Source: CAD feature listing. Evaluate the final solid. Frame: model axes, mm. Face numbers are marked on the shaded views. A direction names the side the tool comes from. Give positions to 0.01 mm unless a question says otherwise; leave off trailing zeros. Loops run counter-clockwise (first coordinate to the right, second up) from the corner with the lowest first, then second, coordinate; pieces in that order, holes last.
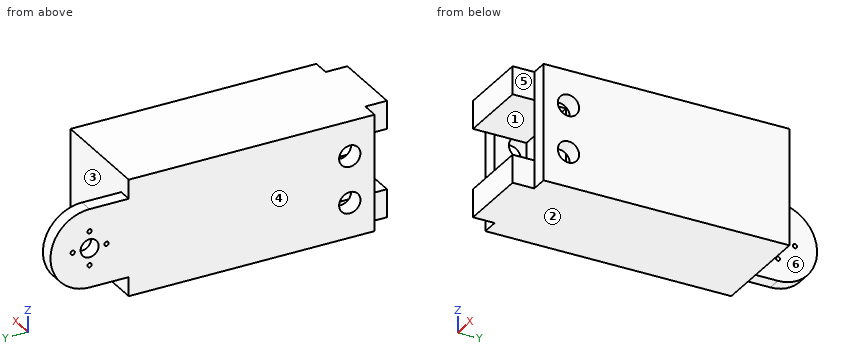
```python
from build123d import *

# Parameters (mm, degrees)
SKETCH1_W               = 50
SKETCH1_H               = 150
BOSS_EXTRUDE1_DEPTH     = 55
CUT_EXTRUDE1_DEPTH      = 168.406690428
CUT_EXTRUDE1_DEPTH_BACK = 45
SKETCH2_R               = 10.25
SKETCH7_R               = 1
SKETCH7_R_2             = 4.25
CUT_EXTRUDE3_DEPTH      = 10
SKETCH8_W               = 55
SKETCH8_H               = 55
SKETCH8_R               = 10.25
BOSS_EXTRUDE2_DEPTH     = 50
SKETCH10_W              = 8
SKETCH10_H              = 10.25
SKETCH10_W_2            = 17
SKETCH10_H_2            = 1
SKETCH10_W_3            = 34
SKETCH10_H_3            = 20
SKETCH10_H_4            = 5
CUT_EXTRUDE4_DEPTH      = 214.717102732
SKETCH11_W              = 34
SKETCH11_H              = 13.25
BOSS_EXTRUDE4_DEPTH     = 25
SKETCH13_W              = 55
SKETCH13_H              = 10
CUT_EXTRUDE5_DEPTH      = 8
SKETCH14_R              = 5.030159043
CUT_EXTRUDE6_DEPTH      = 8
SKETCH15_W              = 34
SKETCH15_H              = 0.25
BOSS_EXTRUDE5_DEPTH     = 13.25
CUT_EXTRUDE7_DEPTH      = 181.416185527
BOSS_EXTRUDE6_START     = 1.5
SKETCH19_R              = 10.25
SKETCH19_R_2            = 1
SKETCH19_R_3            = 4.25
BOSS_EXTRUDE6_DEPTH     = 1.5
CUT_EXTRUDE8_DEPTH      = 184.89467094


with BuildPart() as part:
    # Sketch1 → Boss-Extrude1 (new body)
    with BuildSketch(Plane.XY):
        with Locations((0, -75)):
            Rectangle(SKETCH1_W, SKETCH1_H)
    extrude(amount=-BOSS_EXTRUDE1_DEPTH)

    # Sketch2 → Cut-Extrude1 (cut, two sides: drawn at the far end of the back side and taken through both)
    with BuildSketch(Plane(origin=(25, 0, 0), x_dir=(0, 0, -1), z_dir=(1, 0, 0)).offset(-CUT_EXTRUDE1_DEPTH_BACK)):
        with Locations(Location((27.5, -25, 0), (0, 0, 270))):
            Circle(SKETCH2_R)
    extrude(amount=CUT_EXTRUDE1_DEPTH + CUT_EXTRUDE1_DEPTH_BACK, mode=Mode.SUBTRACT)

    # Sketch7 → Cut-Extrude3 (cut)
    with BuildSketch(Plane(origin=(-20, 0, 0), x_dir=(0, 0, -1), z_dir=(1, 0, 0))):
        with Locations(Location((27.5, -17, 0), (0, 0, 90))):
            Circle(SKETCH7_R)
        with Locations(Location((35.5, -25, 0), (0, 0, 90))):
            Circle(SKETCH7_R)
        with Locations(Location((27.5, -33, 0), (0, 0, 90))):
            Circle(SKETCH7_R)
        with Locations(Location((19.5, -25, 0), (0, 0, 90))):
            Circle(SKETCH7_R)
        with Locations(Location((27.5, -25, 0), (0, 0, 90))):
            Circle(SKETCH7_R_2)
    extrude(amount=-CUT_EXTRUDE3_DEPTH, mode=Mode.SUBTRACT)

    # Sketch8 → Boss-Extrude2 (add)
    with BuildSketch(Plane(origin=(25, 0, 0), x_dir=(0, 0, -1), z_dir=(1, 0, 0))):
        with Locations((27.5, -177.5)):
            Rectangle(SKETCH8_W, SKETCH8_H)
        with Locations(Location((27.5, -180, 0), (0, 0, 90))):
            Circle(SKETCH8_R, mode=Mode.SUBTRACT)
    extrude(amount=-BOSS_EXTRUDE2_DEPTH)

    # Sketch10 → Cut-Extrude4 (cut, through all)
    with BuildSketch(Plane.XY):
        Polygon((-17, -205), (17, -205), (17, -191.25), (0, -191.25), (-17, -191.25), align=None)
        Polygon((-25, -205), (-17, -205), (-17, -191.25), (-17, -190.25), (-25, -190.25), align=None)
        Polygon((17, -191.25), (17, -205), (25, -205), (25, -190.25), (17, -190.25), align=None)
        with Locations((-21, -185.125)):
            Rectangle(SKETCH10_W, SKETCH10_H)
        with Locations((-21, -174.875)):
            Rectangle(SKETCH10_W, SKETCH10_H)
        with Locations((21, -174.875)):
            Rectangle(SKETCH10_W, SKETCH10_H)
        with Locations((21, -185.125)):
            Rectangle(SKETCH10_W, SKETCH10_H)
        with Locations((-8.5, -185.125)):
            Rectangle(SKETCH10_W_2, SKETCH10_H)
        with Locations((8.5, -185.125)):
            Rectangle(SKETCH10_W_2, SKETCH10_H)
        Polygon((0, -180), (17, -180), (17, -169.75), (-17, -169.75), (-17, -180), align=None)
        with Locations((-8.5, -190.75)):
            Rectangle(SKETCH10_W_2, SKETCH10_H_2)
        with Locations((8.5, -190.75)):
            Rectangle(SKETCH10_W_2, SKETCH10_H_2)
        with Locations((0, -154.75)):
            Rectangle(SKETCH10_W_3, SKETCH10_H_3)
        with Locations((0, -167.25)):
            Rectangle(SKETCH10_W_3, SKETCH10_H_4)
    extrude(amount=-CUT_EXTRUDE4_DEPTH, mode=Mode.SUBTRACT)

    # Sketch11 → Boss-Extrude4 (add)
    with BuildSketch(Plane.XZ.offset(144.75)):
        with Locations((0, -6.625)):
            Rectangle(SKETCH11_W, SKETCH11_H)
        with Locations((0, -48.375)):
            Rectangle(SKETCH11_W, SKETCH11_H)
    extrude(amount=BOSS_EXTRUDE4_DEPTH)

    # Sketch13 → Cut-Extrude5 (cut)
    with BuildSketch(Plane(origin=(25, 0, 0), x_dir=(0, 0, -1), z_dir=(1, 0, 0))):
        with Locations((27.5, -164.75)):
            Rectangle(SKETCH13_W, SKETCH13_H)
    cut_extrude5 = extrude(amount=-CUT_EXTRUDE5_DEPTH, mode=Mode.SUBTRACT)

    # Mirror2: Cut-Extrude5 across plane
    add(cut_extrude5.mirror(Plane(origin=(0, 0, 0), x_dir=(0, 0, 1), z_dir=(1, 0, 0))), mode=Mode.SUBTRACT)

    # Sketch14 → Cut-Extrude6 (cut)
    with BuildSketch(Plane(origin=(25, 0, 0), x_dir=(0, 0, -1), z_dir=(1, 0, 0))):
        with Locations(Location((16.5, -148, 0), (0, 0, 90))):
            Circle(SKETCH14_R)
        with Locations(Location((38.5, -148, 0), (0, 0, 90))):
            Circle(SKETCH14_R)
    cut_extrude6 = extrude(amount=-CUT_EXTRUDE6_DEPTH, mode=Mode.SUBTRACT)

    # Mirror3: Cut-Extrude6 across plane
    add(cut_extrude6.mirror(Plane(origin=(0, 0, 0), x_dir=(0, 0, 1), z_dir=(1, 0, 0))), mode=Mode.SUBTRACT)

    # Sketch15 → Boss-Extrude5 (add)
    with BuildSketch(Plane.XY):
        with Locations((0, -169.875)):
            Rectangle(SKETCH15_W, SKETCH15_H)
    boss_extrude5 = extrude(amount=-BOSS_EXTRUDE5_DEPTH)

    # Mirror4: Boss-Extrude5 across plane
    add(boss_extrude5.mirror(Plane.XY.offset(-27.5)))

    # Sketch16 → Cut-Extrude7 (cut, through all)
    with BuildSketch(Plane.XY):
        Polygon((-18.5, 0), (-18.5, -14.75), (-18.5, -35.25), (-18.5, -43.5), (25, -43.5), (25, 0), align=None)
    extrude(amount=-CUT_EXTRUDE7_DEPTH, mode=Mode.SUBTRACT)

    # Sketch19 → Boss-Extrude6 (add)
    with BuildSketch(Plane(origin=(-20, 0, 0), x_dir=(0, 0, -1), z_dir=(1, 0, 0)).offset(BOSS_EXTRUDE6_START)):
        with Locations((27.5, -25)):
            Circle(SKETCH19_R)
        with Locations(Location((27.5, -17, 0), (0, 0, 90))):
            Circle(SKETCH19_R_2, mode=Mode.SUBTRACT)
        with Locations(Location((27.5, -33, 0), (0, 0, 90))):
            Circle(SKETCH19_R_2, mode=Mode.SUBTRACT)
        with Locations(Location((19.5, -25, 0), (0, 0, 90))):
            Circle(SKETCH19_R_2, mode=Mode.SUBTRACT)
        with Locations(Location((35.5, -25, 0), (0, 0, 90))):
            Circle(SKETCH19_R_2, mode=Mode.SUBTRACT)
        with Locations(Location((27.5, -25, 0), (0, 0, 90))):
            Circle(SKETCH19_R_3, mode=Mode.SUBTRACT)
    extrude(amount=-BOSS_EXTRUDE6_DEPTH)

    # Sketch20 → Cut-Extrude8 (cut, through all)
    with BuildSketch(Plane(origin=(-18.5, 0, 0), x_dir=(0, 0, -1), z_dir=(1, 0, 0))):
        with BuildLine():
            Line((0, 0), (0, -43.5))
            Line((0, -43.5), (9, -43.5))
            Line((9, -43.5), (9, -25))
            ThreePointArc((9, -25), (27.5, -6.5), (46, -25))
            Line((46, -25), (46, -43.5))
            Line((46, -43.5), (55, -43.5))
            Line((55, -43.5), (55, 0))
            Line((55, 0), (0, 0))
        make_face()
    extrude(amount=-CUT_EXTRUDE8_DEPTH, mode=Mode.SUBTRACT)


solid = part.part
```
(1) Section B-B, the plane x = -3. Return the cut outline in (y, z).
A:
outline: (-170, -55) - (-43.5, -55) - (-43.5, 0) - (-170, 0) - (-170, -13.25) - (-144.75, -13.25) - (-144.75, -41.75) - (-170, -41.75) - close
(2) Ray query, line 1 along Z through (x, y) = (23, -148); line 2 along Z through (x, y) = (-22.25, -25); line 3 along Y through (x, z) = (-22, -35). Return the intervals inside material, ascending.
A:
line 1: z = -55 to -43.53, -33.47 to -21.53, -11.47 to 0
line 2: z = -46 to -36.5, -34.5 to -31.75, -23.25 to -20.5, -18.5 to -9
line 3: y = -159.75 to -151.61, -144.39 to -25.87, -24.13 to -8.09
(3) Reachability of the marked faces 4, 5 and 6 from +Z, -Z, +X, -X, +Y, -Y: full face, straight path, thin tool, end or side. Return the list, or none.
A:
face 4: +Z, -Z, -X, +Y, -Y
face 5: +Z, -Z, +X, -Y
face 6: +Z, -Z, +X, +Y
(4) Section D-D, the plane x = 22. Return the cut outline in (y, z).
A:
outline: (-159.75, -55) - (-43.5, -55) - (-43.5, 0) - (-159.75, 0) - close; hole circle Ø10.06 at (-148, -38.5); hole circle Ø10.06 at (-148, -16.5)
(5) Mould query, pull axis Z, two halves, no side actions, for the marked faces 1, 2 and 3. Classes: pulls with the +Z half, pulls with the -Z half, needs draft (parallel to the pull), parting line crosses it, or undercut.
A:
face 1: undercut
face 2: pulls with the -Z half
face 3: needs draft
(6) Section A-A, the plane y = -148. Return the cut outline in (x, z), then the cut area to 3 significant figures.
A:
outline: (-25, -55) - (25, -55) - (25, -43.53) - (17, -43.53) - (17, -41.75) - (-17, -41.75) - (-17, -43.53) - (-25, -43.53) - close; (-25, -33.47) - (-17, -33.47) - (-17, -21.53) - (-25, -21.53) - close; (-25, -11.47) - (-17, -11.47) - (-17, -13.25) - (17, -13.25) - (17, -11.47) - (25, -11.47) - (25, 0) - (-25, 0) - close; (17, -33.47) - (25, -33.47) - (25, -21.53) - (17, -21.53) - close
area: 1,460 mm2
(7) Section C-C, the plane z = -38.5. Return the cut outline in (x, y).
A:
outline: (-25, -159.75) - (-17, -159.75) - (-17, -153.03) - (-25, -153.03) - close; (-25, -142.97) - (-17, -142.97) - (-17, -144.75) - (17, -144.75) - (17, -142.97) - (25, -142.97) - (25, -43.5) - (-18.5, -43.5) - (-18.5, -10.13) - (-25, -10.13) - close; (17, -159.75) - (25, -159.75) - (25, -153.03) - (17, -153.03) - close
(8) First-contact query: pin 1 (3 mm diameter, centred on y = -164, z = -51.5, fed in from -X); pin 2 (7 mm diameter, centred on x = -22, y = -32.5, fed in from +Z); pin 3 (2 mm diameter, centred on x = -3.5, z = -34, fed in from +Y). Flat tips, straight axial feed; report the tip coordinate or a pass-through.
A:
pin 1: stops at x = -17
pin 2: stops at z = -9
pin 3: stops at y = -43.5
